For this review, take the finished solid that the model builds, in its own axes (mm). Face numbers are marked on the shaded views. A direction names the side the tool comes from. Coordinates: 2 decimals unless noted, no trailing zeros. Write each loop counter-clockwise with the first axis right and the second up, starting at its lowest first coordinate (ties: lowest second). Pieces come first, ordered by that corner, then holes.
1) We need section A-A on x = 20.5. Write out the cut boundary in (y, z), then the cut area to 3 significant figures.
2) Insertion check: P1, Ø6, axis at x = 54.5, y = -31, coming from the -Z side; P2, Ø6, axis at x = 28.5, y = -15.5, coming from the +Z side; P3, Ø12.5, axis at y = -34.5, z = 39.5, coming from the -X side. Each pin has a flat end and moves straight along its axis. Give the tip position at first contact, or say it passes through.
3) To check wall thickness, follow line 1 along Z through (x, y) = (57, -76); line 2 along X through (y, z) = (-64, 32); line 3 along X through (y, z) = (-60, 45). State the ranges of each line that lie inside material, in increasing order.
4) Mouldability with a two-part tool opening along Z and no side actions: class the marked faces 6, 7 and 8 as pulls with the +Z half, pulls with the -Z half, needs draft (parallel to the pull), parting line crosses it, or undercut.
5) For the marked faces 1, 2, 3, 4 and 5, list the 3-axis set-ups (+Z, -Z, +X, -X, +Y, -Y) from which the entire face can be reached by the end or side of a thin tool; tool diameter is ignored.
6) We need section B-B on y = -8.5. Write out the cut boundary in (x, z).
from build123d import *

# Parameters (mm, degrees)
F0_R        = 44.59812
F1_DEPTH    = 85
F3_DEPTH    = 85.001
F4_T2_ANGLE = 310.1787489512
F4_T4_ANGLE = 310.1787489512


# Not quite as in the source:
# - a fillet or chamfer that OpenCascade refuses, or shapes differently, is made with other operations: its cross-section is extruded or revolved along the edge and cut away or added


with BuildPart() as f1:
    # F0 (on Front) → F1 (new body)
    with BuildSketch(Plane.XZ):
        with Locations((20.5, 21.991262728)):
            Circle(F0_R)
        with BuildLine():
            ThreePointArc((62.0981215365, 21.991262728), (57.0788738932, 2.1824338865), (43.2323802204, -12.8461109515))
            ThreePointArc((43.2323802204, -12.8461109515), (-16.0788738932, 41.8000915695), (62.0981215365, 21.991262728))
        make_face(mode=Mode.SUBTRACT)
        with BuildLine():
            ThreePointArc((62.0981215365, 21.991262728), (-16.0788738932, 41.8000915695), (43.2323802204, -12.8461109515))
            ThreePointArc((43.2323802204, -12.8461109515), (57.0788738932, 2.1824338865), (62.0981215365, 21.991262728))
        make_face()
        with BuildLine():
            Line((48.5, 7.5603930383), (48.5, 1.641262728))
            Line((48.5, 1.641262728), (45.5, 1.641262728))
            Line((45.5, 1.641262728), (45.5, -8.658737272))
            ThreePointArc((45.5, -8.658737272), (44.896697687, -11.0397138467), (43.2323802204, -12.8461109515))
            ThreePointArc((43.2323802204, -12.8461109515), (41.9253300675, -13.4512767031), (40.5, -13.658737272))
            Line((40.5, -13.658737272), (5.8251916537, -13.658737272))
            ThreePointArc((5.8251916537, -13.658737272), (2.8487454964, -12.2827174093), (0, -10.658737272))
            Line((0, -10.658737272), (0, 1.641262728))
            Line((0, 1.641262728), (-7.5, 1.641262728))
            Line((-7.5, 1.641262728), (-7.5, 7.5603930383))
            ThreePointArc((-7.5, 7.5603930383), (-11, 21.991262728), (-7.5, 36.4221324176))
            Line((-7.5, 36.4221324176), (-7.5, 40.641262728))
            Line((-7.5, 40.641262728), (-7.5, 45.641262728))
            Line((-7.5, 45.641262728), (-7.5, 47.641262728))
            ThreePointArc((-7.5, 47.641262728), (-4.5710678119, 54.7123305398), (2.5, 57.641262728))
            Line((2.5, 57.641262728), (38.5, 57.641262728))
            ThreePointArc((38.5, 57.641262728), (45.5710678119, 54.7123305398), (48.5, 47.641262728))
            Line((48.5, 47.641262728), (48.5, 45.641262728))
            Line((48.5, 45.641262728), (48.5, 40.641262728))
            Line((48.5, 40.641262728), (48.5, 36.4221324176))
            ThreePointArc((48.5, 36.4221324176), (52, 21.991262728), (48.5, 7.5603930383))
        make_face(mode=Mode.SUBTRACT)
    extrude(amount=F1_DEPTH)

    # F2 (on face) → F3 (cut, through all)
    with BuildSketch(Plane.XZ.offset(85)):
        with BuildLine():
            Line((5.8251916537, -13.658737272), (5.8251916537, -20.1233702104))
            ThreePointArc((5.8251916537, -20.1233702104), (37.0770201947, -19.4115718247), (60.1846293612, 1.641262728))
            Line((60.1846293612, 1.641262728), (48.5, 1.641262728))
            Line((48.5, 1.641262728), (45.5, 1.641262728))
            Line((45.5, 1.641262728), (45.5, -8.658737272))
            ThreePointArc((45.5, -8.658737272), (44.0355339059, -12.194271178), (40.5, -13.658737272))
            Line((40.5, -13.658737272), (5.8251916537, -13.658737272))
        make_face()
    extrude(amount=-F3_DEPTH, mode=Mode.SUBTRACT)

    # F4: fillet of radius 5 on 2 edges, made by hand

    # F4_s1 → F4_t2 (revolve, cut)
    with BuildSketch(Plane(origin=(20.6066088897, 0, 21.8909083866), x_dir=(0, 1, 0), z_dir=(-0.6854246842, 0, -0.7281435314))):
        with BuildLine():
            ThreePointArc((-85, 39.4517080838), (-83.5355339059, 42.9872419898), (-80, 44.4517080838))
            Line((-80, 44.4517080838), (-85, 44.4517080838))
            Line((-85, 44.4517080838), (-85, 39.4517080838))
        make_face()
    revolve(axis=Axis((20.5, -85, 21.991262728), (0, -1, 0)), revolution_arc=F4_T2_ANGLE, mode=Mode.SUBTRACT)

    # F4_s3 → F4_t4 (revolve, cut)
    with BuildSketch(Plane(origin=(19.2566159931, 0, -1.0396200852), x_dir=(0, 1, 0), z_dir=(0.998545843, 0, -0.0539091767))):
        with BuildLine():
            ThreePointArc((-5, -21.533697897), (-1.4644660941, -20.0692318029), (0, -16.533697897))
            Line((0, -16.533697897), (0, -21.533697897))
            Line((0, -21.533697897), (-5, -21.533697897))
        make_face()
    revolve(axis=Axis((20.5, 0, 21.991262728), (0, 1, 0)), revolution_arc=F4_T4_ANGLE, mode=Mode.SUBTRACT)


solid = f1.part
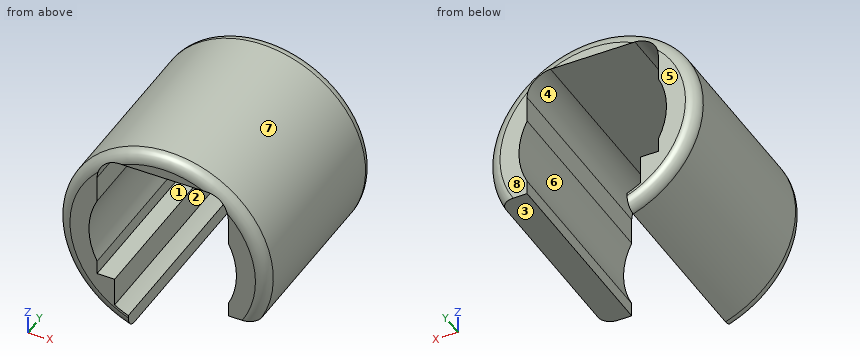
Result:
1. outline: (-85, 57.64) - (0, 57.64) - (0, 61.59) arc R5 ccw to (-5, 66.59) - (-80, 66.59) arc R5 ccw to (-85, 61.59) - close
1. area: 750 mm2
2. P1: stops at z = 1.64
2. P2: stops at z = 66.31
2. P3: stops at x = -22.65
3. line 1: z = 1.64 to 47.62
3. line 2: x = -22.96 to -9.37, 50.37 to 63.96
3. line 3: x = -17.7 to -7.5, 48.5 to 58.7
4. face 6: undercut
4. face 7: parting line crosses it
4. face 8: needs draft
5. face 1: +Y, -Y
5. face 2: +X, +Y, -Y
5. face 3: -Z, +X, +Y, -Y
5. face 4: -Z, +Y, -Y
5. face 5: +Z, -Z, +X, -X, +Y
6. outline: (-7.5, 1.64) - (-7.5, 7.56) arc R31.5 cw to (-7.5, 36.42) - (-7.5, 47.64) arc R10 cw to (2.5, 57.64) - (38.5, 57.64) arc R10 cw to (48.5, 47.64) - (48.5, 36.42) arc R31.5 cw to (48.5, 7.56) - (48.5, 1.64) - (60.18, 1.64) arc R44.6 ccw (long way) to (5.83, -20.12) - (5.83, -13.66) arc R38.55 cw to (0, -10.66) - (0, 1.64) - close
